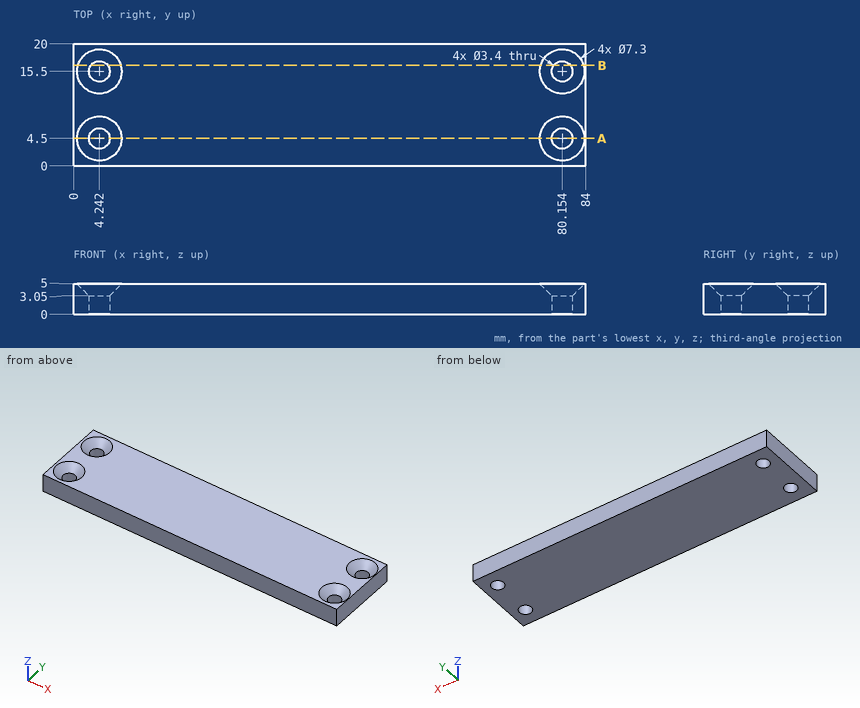
The drawing under review shows one solid part. Ordinate dimensions are in mm from its lowest x, y, z. Give positions to 0.01 mm unless a question says otherwise; leave off trailing zeros. Write each loop counter-clockwise with the first axis right and the second up, starting at its lowest first coordinate (ties: lowest second). Pieces come first, ordered by that corner, then holes. Notation, with made-up numbers: (-32, -17.75) -> (14, -17.75) arc R14 cw to (14, -4.75) -> close; hole circle Ø7 at (-5, 47). An arc over 180 degrees is marked (long way). Use CSV: the item, a comma, the result in double quotes.
Q1. Take a section at B-B, the plane y = 16.5. State how many separate pieces and enclosed holes the cut face has, then the cut area to 3 significant figures.
Conclusion:
separate pieces,"3"
enclosed holes,"0"
area,"384 mm2"
Q2. Take a section at A-A, the plane y = 4.5. Write out the cut boundary in (x, z).
Conclusion:
outline,"(0, 0) -> (2.54, 0) -> (2.54, 3.05) -> (0.59, 5) -> (0, 5) -> close; (5.94, 0) -> (78.45, 0) -> (78.45, 3.05) -> (76.5, 5) -> (7.89, 5) -> (5.94, 3.05) -> close; (81.85, 0) -> (84, 0) -> (84, 5) -> (83.8, 5) -> (81.85, 3.05) -> close"
Q3. To check wall thickness, follow probe 1 along X at (y, z) = (15.5, 0.55); probe 2 along X at (y, z) = (3.5, 2.45) (1 decimal); probe 3 along Z at (x, y) = (7, 15.5). State the ranges of each line that lie inside material, in increasing order. Write a range as [from, to].
Conclusion:
probe 1,"[0, 2.54], [5.94, 78.45], [81.85, 84]"
probe 2,"[0, 2.9], [5.6, 78.8], [81.5, 84]"
probe 3,"[0, 4.11]"
